from build123d import *

# Parameters (mm, degrees)
SKETCH_2_R   = 5
SKETCH_2_R_2 = 4


with BuildPart() as part:
    # По траектории1: sweep along a path in Эскиз1
    with BuildLine(Plane.XY) as sweep_1_path:
        ThreePointArc((0, 12.5), (-12.5, 0), (0, -12.5))
    # Эскиз2 → По траектории1 (sweep)
    with BuildSketch(Plane(origin=(0, 0, 0), x_dir=(0, 0, -1), z_dir=(1, 0, 0))):
        with Locations((0, 12.5)):
            Circle(SKETCH_2_R)
        with Locations((0, 12.5)):
            Circle(SKETCH_2_R_2, mode=Mode.SUBTRACT)
    sweep(path=sweep_1_path.line)

    # Эскиз3 → Повернуть1 (revolve)
    with BuildSketch(Plane.XY, mode=Mode.PRIVATE) as revolve_1_sk:
        Polygon((4, 19.5), (0, 17.5), (0, 16.5), (4, 16.5), align=None)
    revolve(revolve_1_sk.sketch.rotate(Axis((-2.915316987, 12.5, 0), (1, 0, 0)), 270), axis=Axis((-2.915316987, 12.5, 0), (1, 0, 0)))

    # Эскиз5 → Повернуть2 (revolve)
    with BuildSketch(Plane.XY, mode=Mode.PRIVATE) as revolve_2_sk:
        Polygon((4, -5.5), (0, -7.5), (0, -8.5), (4, -8.5), align=None)
    revolve(revolve_2_sk.sketch.rotate(Axis((-1.97650581, -12.5, 0), (1, 0, 0)), 180), axis=Axis((-1.97650581, -12.5, 0), (1, 0, 0)))


solid = part.part
Model file for the job. Use its own axes, mm. A direction names the side the tool comes from. Give positions to 0.01 mm unless a question says otherwise; leave off trailing zeros. Order: outer loops, then holes, each group sorted by start corner. A loop starts at its lowest first (then second) coordinate and runs counter-clockwise, first axis right, second up. Notation, with made-up numbers: M -25.75,18.5 L 29.25,18.5 A36 cw 29.25,54.5 Z; hole C 86,85.25 d2. An arc over 180 degrees is marked long. Put each result on its own line as item: value. Start each with the question number.
(1) Pin check, flat tips, straight feed: pin 1 Ø2 at (y, z) = (10, -4.5) entering from -X; pin 2 Ø1 at (x, z) = (-6, 3) entering from -Y; pin 3 Ø6 at (x, z) = (-14, -2) entering from -Y. Stop position of each tip, or through.
(2) Drill centre lines: L1, parallel to X at y = -7.5, z = -3; L2, parallel to X at y = -4.5, z = -3.5; L3, parallel to Z at x = -8.5, y = 8. Where is each one in solid material? Low to high. Write a range as [from, to].
(3) Pull direction Z, two halves, no side cores. Call faces 1 (the face through (4, 9, 3)), 2 (the face through (0.194, 7.524, 1.105)), 3 (the face through (2.028, 16.466, 0.521)): released by +Z, released by -Z, zero draft, split by the parting line, or undercut.
(4) Tool access for faces 4 (the face through (4, -9, 3)), 5 (the face through (2, -9.3, 2.4)), 6 (the face through (0.194, -17.208, 1.952)): list every direction of +Z, -Z, +X, -X, +Y, -Y with a clear straight run to the whole face (end or side of a thin tool).
(5) Band-saw the part on B-B on x = 2. Give the cut face in (y, z), then the cut area to 3 significant figures.
(6) Band-saw the part on C-C on x = -4. Count the separate pieces of the cut face and the enclosed holes in it, then the cut area to 3 significant figures.
(7) Band-saw the part on A-A on z = 0. Give the cut face in (x, y).
Results below:
1. pin 1: stops at x = -12.79
1. pin 2: stops at y = -15.78
1. pin 3: stops at y = -13.34
2. L1: x = [-14.7, -13.16], [-6.39, -4], [1.66, 4]
2. L2: x = [-15.43, -13.72], [-9.56, -7.71]
2. L3: z = [-4.93, -3.91], [3.91, 4.93]
3. face 1: zero draft
3. face 2: split by the parting line
3. face 3: undercut
4. face 4: +Z, -Z, +X, +Y, -Y
4. face 5: +X
4. face 6: none
5. outline: C -12.5,0 d12; C 12.5,0 d12; hole C -12.5,0 d8; hole C 12.5,0 d8
5. area: 126 mm2
6. separate pieces: 2
6. enclosed holes: 2
6. area: 60.7 mm2
7. outline: M 0,-17.5 L 4,-19.5 L 4,-16.5 L 0,-16.5 A16.5 cw 0,16.5 L 4,16.5 L 4,19.5 L 0,17.5 A17.5 ccw Z; M 0,-8.5 L 4,-8.5 L 4,-5.5 L 0,-7.5 A7.5 cw 0,7.5 L 4,5.5 L 4,8.5 L 0,8.5 A8.5 ccw Z
